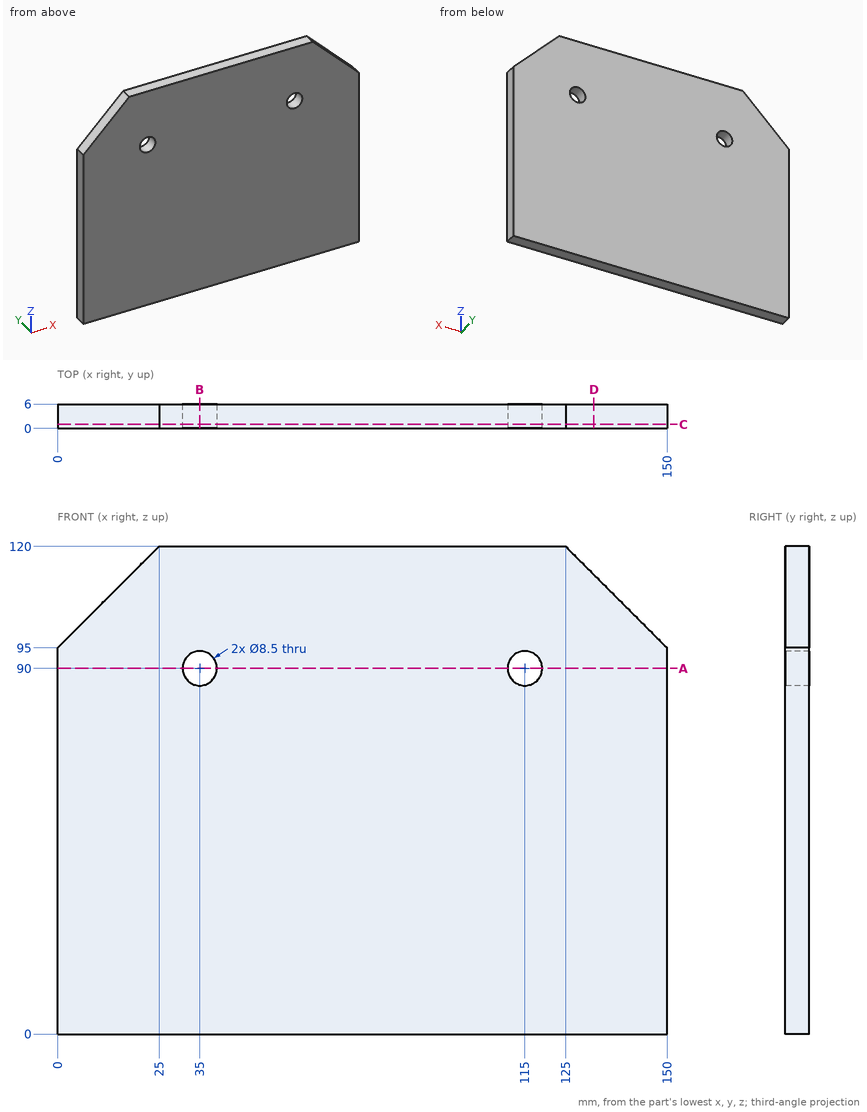
Answer from the drawing. Dimensions are ordinates in mm from the lowest x, y and z of the part. Give positions to 0.01 mm unless a question says otherwise; leave off trailing zeros. Order: outer loops, then holes, each group sorted by start corner. A loop starts at its lowest first (then second) coordinate and runs counter-clockwise, first axis right, second up. Notation, with made-up numbers: (44.25, 24.5) -> (59.25, 24.5) arc R23 cw to (59.25, 35.5) -> close; hole circle Ø4 at (42, 61). An arc over 180 degrees is marked (long way). One line per item, written item: value.
Item 1: Find section D-D, the plane x = 132. Give the vertices of the cut face in (y, z).
Answer sheet:
outline: (0, 0) -> (6, 0) -> (6, 113) -> (0, 113) -> close
Item 2: Find section A-A, the plane z = 90. Give the vertices of the cut face in (x, y), plus the area to 3 significant figures.
Answer sheet:
outline: (0, 0) -> (30.75, 0) -> (30.75, 6) -> (0, 6) -> close; (39.25, 0) -> (110.75, 0) -> (110.75, 6) -> (39.25, 6) -> close; (119.25, 0) -> (150, 0) -> (150, 6) -> (119.25, 6) -> close
area: 798 mm²
Item 3: Find section B-B, the plane x = 35. Give the vertices of the cut face in (y, z).
Answer sheet:
outline: (0, 0) -> (6, 0) -> (6, 85.75) -> (0, 85.75) -> close; (0, 94.25) -> (6, 94.25) -> (6, 120) -> (0, 120) -> close
Item 4: Find section C-C, the plane y = 1. Give the vertices of the cut face in (x, z).
Answer sheet:
outline: (0, 0) -> (150, 0) -> (150, 95) -> (125, 120) -> (25, 120) -> (0, 95) -> close; hole circle Ø8.5 at (35, 90); hole circle Ø8.5 at (115, 90)
Item 5: Straight lines are drawn through the part: probe 1 along Z at (x, y) = (115, 3); probe 2 along Z at (x, y) = (113, 2); probe 3 along X at (y, z) = (1, 114.5). For each, find the intervals that lie inside material, in ascending order.
Answer sheet:
probe 1: 0 to 85.75, 94.25 to 120
probe 2: 0 to 86.25, 93.75 to 120
probe 3: 19.5 to 130.5
